CAD build for the part. Positions are in the model's coordinates, mm. Coordinates: 2 decimals unless noted, no trailing zeros. Write each loop counter-clockwise with the first axis right and the second up, starting at its lowest first coordinate (ties: lowest second). Pieces come first, ordered by that corner, then holes. Notation, with made-up numbers: (8.5, -26.75) - (34.5, -26.75) arc R20 ccw to (34.5, -9.75) - close; hole circle Ø1 at (34.5, -19). An arc over 180 degrees is marked (long way). One line per question, with ' | ' between items. Start each with the question number.
1. Band-saw the part on B-B, the plane z = 1.75. Write the cut outline in (x, y).
2. Probe line 1 (Y direction, x = -52, z = 7.5); line 2 (Y direction, x = 95, z = 6.75); line 3 (X direction, y = 68, z = 7). List the from-to ranges inside material, lowest first.
3. Band-saw the part on C-C, the plane x = -67. Write the cut outline in (y, z).
4. Flat gauge pins, fed straight in: P1, Ø4, axis at x = 73.5, z = 1.5, coming from the +Y side (3 decimals); P2, Ø2.5, axis at x = -95, y = 22, coming from the +Z side; P3, Ø1.5, axis at y = 41, z = 4.5, coming from the -X side. Where does each tip first touch, or does it go through?
5. Band-saw the part on D-D, the plane y = -48. Write the cut outline in (x, z), then the cut area to 3 significant figures.
6. Band-saw the part on A-A, the plane y = 23. Write the cut outline in (x, z).
from build123d import *

# Parameters (mm, degrees)
BOSS_EXTRUDE2_DEPTH = 15
SKETCH2_W           = 3
SKETCH2_H           = 20
CUT_EXTRUDE2_DEPTH  = 10
SKETCH4_W           = 3
SKETCH4_H           = 20
BOSS_EXTRUDE5_DEPTH = 10
CUT_EXTRUDE3_DEPTH  = 5
SKETCH6_R           = 2.5
CUT_EXTRUDE4_DEPTH  = 6


with BuildPart() as part:
    # Sketch1 → Boss-Extrude2 (new body)
    with BuildSketch(Plane.XY):
        Polygon((-52, 100), (52, 100), (72, 95), (72, 33), (100, 28), (100, -28), (72, -33), (72, -95), (52, -100), (-52, -100), (-72, -95), (-72, -33), (-100, -28), (-100, 28), (-72, 33), (-72, 95.107401563), align=None)
    extrude(amount=BOSS_EXTRUDE2_DEPTH)

    # Sketch2 → Cut-Extrude2 (cut)
    with BuildSketch(Plane.XY.offset(15)):
        with Locations((-69.5, 80.352031484)):
            Rectangle(SKETCH2_W, SKETCH2_H)
        with Locations((-69.5, 43)):
            Rectangle(SKETCH2_W, SKETCH2_H)
    extrude(amount=-CUT_EXTRUDE2_DEPTH, mode=Mode.SUBTRACT)

    # Sketch4 → Boss-Extrude5 (add)
    with BuildSketch(Plane.XY.offset(15)):
        Polygon((-71, 90.352031484), (-68, 90.352031484), (-68, 70.352031484), (-69.5, 70.352031484), (-71, 70.352031484), align=None)
        with Locations((-69.5, 43)):
            Rectangle(SKETCH4_W, SKETCH4_H)
    extrude(amount=-BOSS_EXTRUDE5_DEPTH)

    # Sketch5 → Cut-Extrude3 (cut)
    with BuildSketch(Plane.XY.offset(15)):
        Polygon((-72, 95.107401563), (-72, 33), (-100, 28), (-100, -28), (-72, -33), (-72, -95), (-52, -100), (52, -100), (72, -95), (72, -33), (100, -28), (100, 28), (72, 33), (72, 95), (52, 100), (-52, 100), align=None)
    extrude(amount=-CUT_EXTRUDE3_DEPTH, mode=Mode.SUBTRACT)

    # Sketch6 → Cut-Extrude4 (cut)
    with BuildSketch(Plane.XY.offset(10)):
        with Locations((-52, 95.107401563)):
            Circle(SKETCH6_R)
        with Locations((-52, -95)):
            Circle(SKETCH6_R)
        with Locations((-67, -33)):
            Circle(SKETCH6_R)
        with Locations((-67, 33)):
            Circle(SKETCH6_R)
        with Locations((-95, 23)):
            Circle(SKETCH6_R)
        with Locations((-95, -23)):
            Circle(SKETCH6_R)
        with Locations(Location((95, -23, 0), (0, 0, 180))):
            Circle(SKETCH6_R)
        with Locations(Location((95, 23, 0), (0, 0, 180))):
            Circle(SKETCH6_R)
        with Locations(Location((67, 33, 0), (0, 0, 180))):
            Circle(SKETCH6_R)
        with Locations(Location((67, -33, 0), (0, 0, 180))):
            Circle(SKETCH6_R)
        with Locations(Location((52, -95, 0), (0, 0, 180))):
            Circle(SKETCH6_R)
        with Locations(Location((52, 95.107401563, 0), (0, 0, 180))):
            Circle(SKETCH6_R)
    extrude(amount=-CUT_EXTRUDE4_DEPTH, mode=Mode.SUBTRACT)


solid = part.part
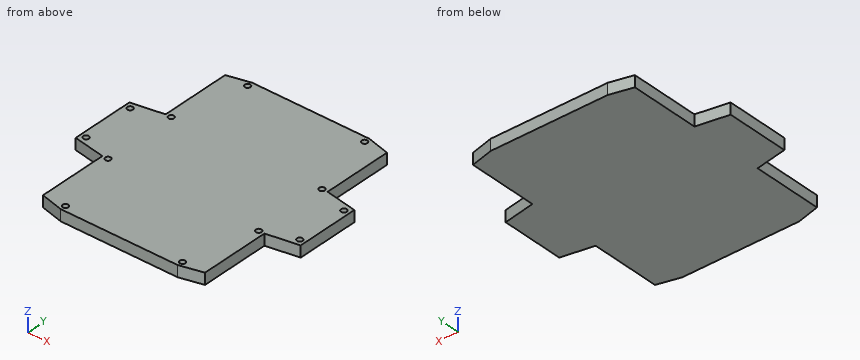
Filled in:
1) outline: (-100, -28) - (-72, -33) - (-72, -95) - (-52, -100) - (52, -100) - (72, -95) - (72, -33) - (100, -28) - (100, 28) - (72, 33) - (72, 95) - (52, 100) - (-52, 100) - (-72, 95.11) - (-72, 33) - (-100, 28) - close
2) line 1: y = -100 to -97.5, -92.5 to 92.61, 97.61 to 100 | line 2: y = -28.89 to -25.5, -20.5 to 20.5, 25.5 to 28.89 | line 3: x = -72 to 72
3) outline: (-96.25, 0) - (96.33, 0) - (96.33, 10) - (35.5, 10) - (35.5, 4) - (30.5, 4) - (30.5, 10) - (-30.5, 10) - (-30.5, 4) - (-35.5, 4) - (-35.5, 10) - (-96.25, 10) - close
4) P1: stops at y = 95.125 | P2: stops at z = 4 | P3: stops at x = -72
5) outline: (-72, 0) - (72, 0) - (72, 10) - (-72, 10) - close | area: 1,440 mm²
6) outline: (-100, 0) - (100, 0) - (100, 10) - (97.5, 10) - (97.5, 4) - (92.5, 4) - (92.5, 10) - (-92.5, 10) - (-92.5, 4) - (-97.5, 4) - (-97.5, 10) - (-100, 10) - close
